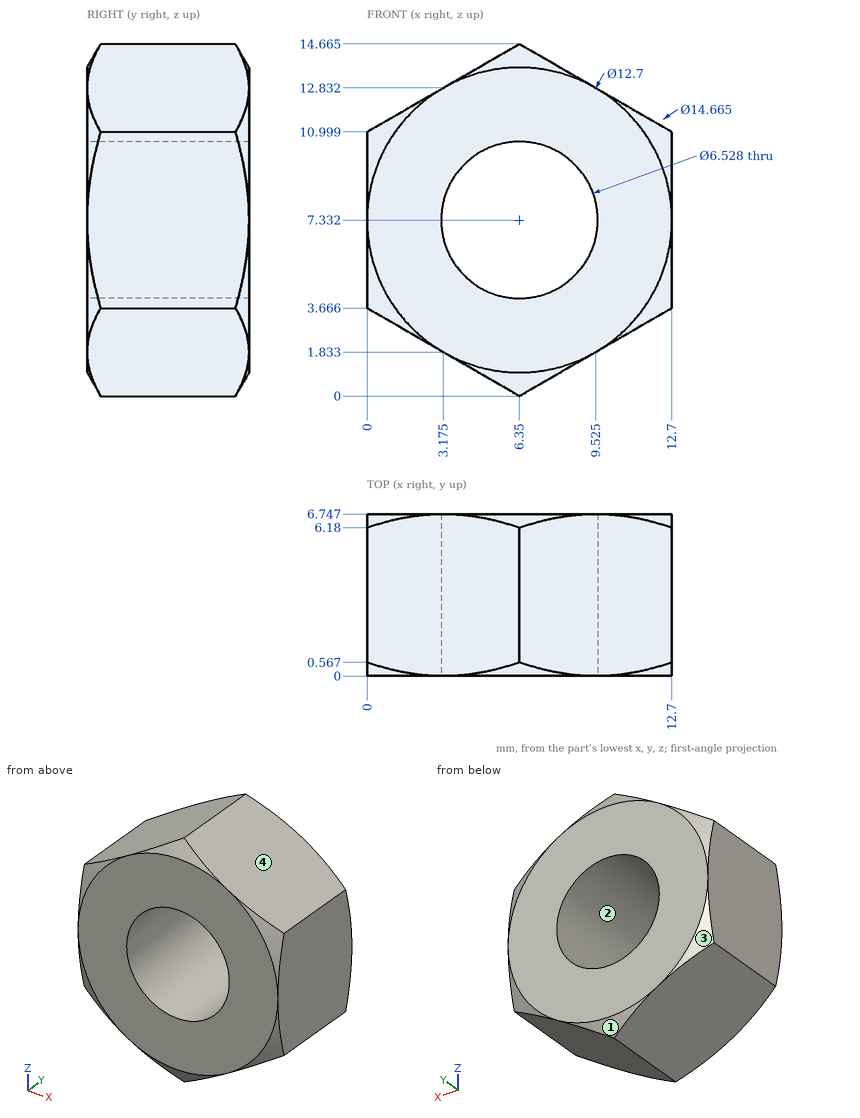
The figure shows three views and two pictorial views of one solid part (mm, origin at its lowest corner). Answer the questions. Coordinates: 2 decimals unless noted, no trailing zeros.
1) Flat-ended cylindrical pins translate along their axes: pin 1 Ø4 at (x, y) = (2.5, 4) entering from -Z; pin 2 Ø3 at (x, y) = (10, 3.5) entering from -Z; pin 3 Ø1 at (x, y) = (9.5, 1) entering from +Z (1 decimal). Find the tip coordinate at first contact, or state that the pin passes through.
2) Determine the mould class of the marked faces 1, 2, 3 and 4 for opening direction X: pulls with the +X half, pulls with the -X half, needs draft (parallel to the pull), parting line crosses it, or undercut.
3) Find the intervals of material crossed by L1, parallel to X at y = 5.25, z = 7; L2, parallel to X at y = 5, z = 8.25; L3, parallel to Z at x = 5, y = 4.5 (1 decimal), in increasing order.
Values:
1. pin 1: stops at z = 1.07
1. pin 2: stops at z = 1.24
1. pin 3: stops at z = 13.1
2. face 1: parting line crosses it
2. face 2: undercut
2. face 3: pulls with the -X half
2. face 4: pulls with the +X half
3. L1: x = 0 to 3.1, 9.6 to 12.7
3. L2: x = 0 to 3.22, 9.48 to 12.7
3. L3: z = 0.8 to 4.4, 10.3 to 13.9
